Design review of the part built by this model. Coordinates are the model's own, in mm. Face numbers are marked on the shaded views. A direction names the side the tool comes from. Round coordinates to 2 decimals unless told otherwise and drop trailing zeros. Loops run counter-clockwise (first coordinate to the right, second up) from the corner with the lowest first, then second, coordinate; pieces in that order, holes last. Notation, with made-up numbers: M -40,-16 L 3,-16 A34 cw 3,18 Z; hole C 48,54 d2. An arc over 180 degrees is marked long. One line per item, written item: value. Start each with the question number.
Item 1: We need section D-D (y = -20.5). Write out the cut boundary in (x, z) (3 decimals), then the cut area to 3 significant figures.
Item 2: We need section A-A (z = -1.25). Write out the cut boundary in (x, y).
Item 3: Clearance check with flat-ended pins moving along their axes: pin 1 (5 mm diameter, centred on x = -11.5, z = -11, fed in from +Y); pin 2 (2 mm diameter, centred on x = 15.24, z = -11.625, fed in from +Y). State where each tip first meets the part, or that it passes through.
Item 4: We need section C-C (x = 11). Write out the cut boundary in (y, z), then the cut area to 3 significant figures.
Item 5: For the marked faces 1, 2 and 3, list the 3-axis set-ups (+Z, -Z, +X, -X, +Y, -Y) from which the entire face can be reached by the end or side of a thin tool; tool diameter is ignored.
Item 6: We need section B-B (z = -8). Write out the cut boundary in (x, y).
Item 7: Mouldability with a two-part tool opening along Y and no side actions: class the marked faces 4, 5 and 6 as released by +Y, released by -Y, zero draft, split by the parting line, or undercut.
Item 8: For line 1 along Y through (x, z) = (-6.35, 0.7); line 2 along X through (y, z) = (-17, -8.5); line 3 along Y through (x, z) = (-11, 1.75), list the stretches that pass through material, from the lowest coordinate up.
from build123d import *
from OCP.BRepFilletAPI import BRepFilletAPI_MakeChamfer

# Parameters (mm, degrees)
SKETCH_1_W          = 38.1
SKETCH_1_H          = 48
EXTRUDE_1_DEPTH     = 3
SKETCH_2_R          = 0.4
CUT_EXTRUDE_1_DEPTH = 31.78802527
SKETCH_3_W          = 38.1
SKETCH_3_H          = 15
EXTRUDE_2_DEPTH     = 17
SKETCH_4_W          = 2.75
SKETCH_4_H          = 2.75
CUT_EXTRUDE_2_DEPTH = 4
CHAMFER_1_SIZE      = 1
CHAMFER_1_SIZE_2    = 4
SKETCH_5_R          = 0.8
CUT_EXTRUDE_5_DEPTH = 55.36821222
SKETCH_6_W          = 38.1
SKETCH_6_H          = 11
CUT_EXTRUDE_6_DEPTH = 10
CUT_EXTRUDE_7_REACH = 34.232
SKETCH_8_W          = 1.6
SKETCH_8_H          = 6.622641265


with BuildPart() as part:
    # 草圖1 → 填料-伸長1 (new body)
    with BuildSketch(Plane.XY):
        Rectangle(SKETCH_1_W, SKETCH_1_H)
    extrude(amount=EXTRUDE_1_DEPTH)

    # 草圖2 → 除料-伸長1 (cut, through all)
    with BuildSketch(Plane.XY.offset(3)):
        with Locations((-16.51, 19)):
            Circle(SKETCH_2_R)
        with Locations((-13.97, 19)):
            Circle(SKETCH_2_R)
        with Locations((-6.35, 19)):
            Circle(SKETCH_2_R)
        with Locations((-3.81, 19)):
            Circle(SKETCH_2_R)
        with Locations((3.81, 19)):
            Circle(SKETCH_2_R)
        with Locations((6.35, 19)):
            Circle(SKETCH_2_R)
        with Locations((13.97, 19)):
            Circle(SKETCH_2_R)
        with Locations((16.51, 19)):
            Circle(SKETCH_2_R)
    extrude(amount=-CUT_EXTRUDE_1_DEPTH, mode=Mode.SUBTRACT)

    # 草圖3 → 填料-伸長2 (add)
    with BuildSketch(Plane(origin=(0, 0, 0), x_dir=(-1, 0, 0), z_dir=(0, 0, -1))):
        with Locations((0, -16.5)):
            Rectangle(SKETCH_3_W, SKETCH_3_H)
    extrude(amount=EXTRUDE_2_DEPTH)

    # 草圖4 → 除料-伸長2 (cut)
    with BuildSketch(Plane(origin=(0, -9, 0), x_dir=(1, 0, 0), z_dir=(0, 1, 0))):
        with Locations((-15.24, 11.625)):
            Rectangle(SKETCH_4_W, SKETCH_4_H)
        with Locations((-5.08, 11.625)):
            Rectangle(SKETCH_4_W, SKETCH_4_H)
        with Locations((5.08, 11.625)):
            Rectangle(SKETCH_4_W, SKETCH_4_H)
        with Locations((15.24, 11.625)):
            Rectangle(SKETCH_4_W, SKETCH_4_H)
    extrude(amount=-CUT_EXTRUDE_2_DEPTH, mode=Mode.SUBTRACT)

    # 導角1
    chamfer_1_edges_1 = [part.edges().sort_by_distance(p)[0] for p in [
        (-15.24, -9, -13),
    ]]
    chamfer_1_side_1 = [part.faces().sort_by_distance(p)[0] for p in [
        (-15.24, -9, -13.02),
    ]]
    chamfer_1_edges_2 = [part.edges().sort_by_distance(p)[0] for p in [
        (-13.865, -9, -11.625),
    ]]
    chamfer_1_side_2 = [part.faces().sort_by_distance(p)[0] for p in [
        (-13.845, -9, -11.625),
    ]]
    chamfer_1_edges_3 = [part.edges().sort_by_distance(p)[0] for p in [
        (-16.615, -9, -11.625),
    ]]
    chamfer_1_side_3 = [part.faces().sort_by_distance(p)[0] for p in [
        (-16.635, -9, -11.625),
    ]]
    chamfer_1_edges_4 = [part.edges().sort_by_distance(p)[0] for p in [
        (-15.24, -9, -10.25),
    ]]
    chamfer_1_side_4 = [part.faces().sort_by_distance(p)[0] for p in [
        (-15.24, -9, -10.23),
    ]]
    chamfer_1_edges_5 = [part.edges().sort_by_distance(p)[0] for p in [
        (15.24, -9, -10.25),
    ]]
    chamfer_1_side_5 = [part.faces().sort_by_distance(p)[0] for p in [
        (15.24, -9, -10.23),
    ]]
    chamfer_1_edges_6 = [part.edges().sort_by_distance(p)[0] for p in [
        (13.865, -9, -11.625),
    ]]
    chamfer_1_side_6 = [part.faces().sort_by_distance(p)[0] for p in [
        (13.845, -9, -11.625),
    ]]
    chamfer_1_edges_7 = [part.edges().sort_by_distance(p)[0] for p in [
        (16.615, -9, -11.625),
    ]]
    chamfer_1_side_7 = [part.faces().sort_by_distance(p)[0] for p in [
        (16.635, -9, -11.625),
    ]]
    chamfer_1_edges_8 = [part.edges().sort_by_distance(p)[0] for p in [
        (15.24, -9, -13),
    ]]
    chamfer_1_side_8 = [part.faces().sort_by_distance(p)[0] for p in [
        (15.24, -9, -13.02),
    ]]
    chamfer_1_edges_9 = [part.edges().sort_by_distance(p)[0] for p in [
        (5.08, -9, -10.25),
    ]]
    chamfer_1_side_9 = [part.faces().sort_by_distance(p)[0] for p in [
        (5.08, -9, -10.23),
    ]]
    chamfer_1_edges_10 = [part.edges().sort_by_distance(p)[0] for p in [
        (6.455, -9, -11.625),
    ]]
    chamfer_1_side_10 = [part.faces().sort_by_distance(p)[0] for p in [
        (6.475, -9, -11.625),
    ]]
    chamfer_1_edges_11 = [part.edges().sort_by_distance(p)[0] for p in [
        (5.08, -9, -13),
    ]]
    chamfer_1_side_11 = [part.faces().sort_by_distance(p)[0] for p in [
        (5.08, -9, -13.02),
    ]]
    chamfer_1_edges_12 = [part.edges().sort_by_distance(p)[0] for p in [
        (3.705, -9, -11.625),
    ]]
    chamfer_1_side_12 = [part.faces().sort_by_distance(p)[0] for p in [
        (3.685, -9, -11.625),
    ]]
    chamfer_1_edges_13 = [part.edges().sort_by_distance(p)[0] for p in [
        (-5.08, -9, -10.25),
    ]]
    chamfer_1_side_13 = [part.faces().sort_by_distance(p)[0] for p in [
        (-5.08, -9, -10.23),
    ]]
    chamfer_1_edges_14 = [part.edges().sort_by_distance(p)[0] for p in [
        (-6.455, -9, -11.625),
    ]]
    chamfer_1_side_14 = [part.faces().sort_by_distance(p)[0] for p in [
        (-6.475, -9, -11.625),
    ]]
    chamfer_1_edges_15 = [part.edges().sort_by_distance(p)[0] for p in [
        (-5.08, -9, -13),
    ]]
    chamfer_1_side_15 = [part.faces().sort_by_distance(p)[0] for p in [
        (-5.08, -9, -13.02),
    ]]
    chamfer_1_edges_16 = [part.edges().sort_by_distance(p)[0] for p in [
        (-3.705, -9, -11.625),
    ]]
    chamfer_1_side_16 = [part.faces().sort_by_distance(p)[0] for p in [
        (-3.685, -9, -11.625),
    ]]
    chamfer_1 = BRepFilletAPI_MakeChamfer(part.part.solid().wrapped)
    for e in chamfer_1_edges_1:
        chamfer_1.Add(CHAMFER_1_SIZE - 0.0001, CHAMFER_1_SIZE_2 - 0.0001, e.wrapped, chamfer_1_side_1[0].wrapped)
    for e in chamfer_1_edges_2:
        chamfer_1.Add(CHAMFER_1_SIZE - 0.0001, CHAMFER_1_SIZE_2 - 0.0001, e.wrapped, chamfer_1_side_2[0].wrapped)
    for e in chamfer_1_edges_3:
        chamfer_1.Add(CHAMFER_1_SIZE - 0.0001, CHAMFER_1_SIZE_2 - 0.0001, e.wrapped, chamfer_1_side_3[0].wrapped)
    for e in chamfer_1_edges_4:
        chamfer_1.Add(CHAMFER_1_SIZE - 0.0001, CHAMFER_1_SIZE_2 - 0.0001, e.wrapped, chamfer_1_side_4[0].wrapped)
    for e in chamfer_1_edges_5:
        chamfer_1.Add(CHAMFER_1_SIZE - 0.0001, CHAMFER_1_SIZE_2 - 0.0001, e.wrapped, chamfer_1_side_5[0].wrapped)
    for e in chamfer_1_edges_6:
        chamfer_1.Add(CHAMFER_1_SIZE - 0.0001, CHAMFER_1_SIZE_2 - 0.0001, e.wrapped, chamfer_1_side_6[0].wrapped)
    for e in chamfer_1_edges_7:
        chamfer_1.Add(CHAMFER_1_SIZE - 0.0001, CHAMFER_1_SIZE_2 - 0.0001, e.wrapped, chamfer_1_side_7[0].wrapped)
    for e in chamfer_1_edges_8:
        chamfer_1.Add(CHAMFER_1_SIZE - 0.0001, CHAMFER_1_SIZE_2 - 0.0001, e.wrapped, chamfer_1_side_8[0].wrapped)
    for e in chamfer_1_edges_9:
        chamfer_1.Add(CHAMFER_1_SIZE - 0.0001, CHAMFER_1_SIZE_2 - 0.0001, e.wrapped, chamfer_1_side_9[0].wrapped)
    for e in chamfer_1_edges_10:
        chamfer_1.Add(CHAMFER_1_SIZE - 0.0001, CHAMFER_1_SIZE_2 - 0.0001, e.wrapped, chamfer_1_side_10[0].wrapped)
    for e in chamfer_1_edges_11:
        chamfer_1.Add(CHAMFER_1_SIZE - 0.0001, CHAMFER_1_SIZE_2 - 0.0001, e.wrapped, chamfer_1_side_11[0].wrapped)
    for e in chamfer_1_edges_12:
        chamfer_1.Add(CHAMFER_1_SIZE - 0.0001, CHAMFER_1_SIZE_2 - 0.0001, e.wrapped, chamfer_1_side_12[0].wrapped)
    for e in chamfer_1_edges_13:
        chamfer_1.Add(CHAMFER_1_SIZE - 0.0001, CHAMFER_1_SIZE_2 - 0.0001, e.wrapped, chamfer_1_side_13[0].wrapped)
    for e in chamfer_1_edges_14:
        chamfer_1.Add(CHAMFER_1_SIZE - 0.0001, CHAMFER_1_SIZE_2 - 0.0001, e.wrapped, chamfer_1_side_14[0].wrapped)
    for e in chamfer_1_edges_15:
        chamfer_1.Add(CHAMFER_1_SIZE - 0.0001, CHAMFER_1_SIZE_2 - 0.0001, e.wrapped, chamfer_1_side_15[0].wrapped)
    for e in chamfer_1_edges_16:
        chamfer_1.Add(CHAMFER_1_SIZE - 0.0001, CHAMFER_1_SIZE_2 - 0.0001, e.wrapped, chamfer_1_side_16[0].wrapped)
    add(Compound.cast(chamfer_1.Shape()), mode=Mode.REPLACE)  # a hair under: the kernel refuses the full size

    # 草圖5 → 除料-伸長5 (cut, through all)
    with BuildSketch(Plane.XZ.offset(24)):
        with Locations(Location((-15.24, -11.625, 0), (0, 0, 270))):
            Circle(SKETCH_5_R)
        with Locations(Location((-5.08, -11.625, 0), (0, 0, 270))):
            Circle(SKETCH_5_R)
        with Locations(Location((5.08, -11.625, 0), (0, 0, 270))):
            Circle(SKETCH_5_R)
        with Locations(Location((15.24, -11.625, 0), (0, 0, 270))):
            Circle(SKETCH_5_R)
    extrude(amount=-CUT_EXTRUDE_5_DEPTH, mode=Mode.SUBTRACT)

    # 草圖6 → 除料-伸長6 (cut)
    with BuildSketch(Plane.XY.offset(3)):
        with Locations((0, -16.5)):
            Rectangle(SKETCH_6_W, SKETCH_6_H)
    extrude(amount=-CUT_EXTRUDE_6_DEPTH, mode=Mode.SUBTRACT)

    # 草圖8 → 除料-伸長7 (cut, up to next)
    with BuildSketch(Plane.XY.offset(-7), mode=Mode.PRIVATE) as cut_extrude_7_sk1:
        with Locations((-15.24, -18.688679368)):
            Rectangle(SKETCH_8_W, SKETCH_8_H)
    cut_extrude_7_tool1 = extrude(cut_extrude_7_sk1.sketch, amount=-CUT_EXTRUDE_7_REACH, mode=Mode.PRIVATE) & part.part
    # 草圖8 → 除料-伸長7 (cut, up to next)
    with BuildSketch(Plane.XY.offset(-7), mode=Mode.PRIVATE) as cut_extrude_7_sk2:
        with Locations((-5.08, -18.688679368)):
            Rectangle(SKETCH_8_W, SKETCH_8_H)
    cut_extrude_7_tool2 = extrude(cut_extrude_7_sk2.sketch, amount=-CUT_EXTRUDE_7_REACH, mode=Mode.PRIVATE) & part.part
    # 草圖8 → 除料-伸長7 (cut, up to next)
    with BuildSketch(Plane.XY.offset(-7), mode=Mode.PRIVATE) as cut_extrude_7_sk3:
        with Locations((5.08, -18.688679368)):
            Rectangle(SKETCH_8_W, SKETCH_8_H)
    cut_extrude_7_tool3 = extrude(cut_extrude_7_sk3.sketch, amount=-CUT_EXTRUDE_7_REACH, mode=Mode.PRIVATE) & part.part
    # 草圖8 → 除料-伸長7 (cut, up to next)
    with BuildSketch(Plane.XY.offset(-7), mode=Mode.PRIVATE) as cut_extrude_7_sk4:
        with Locations((15.24, -18.688679368)):
            Rectangle(SKETCH_8_W, SKETCH_8_H)
    cut_extrude_7_tool4 = extrude(cut_extrude_7_sk4.sketch, amount=-CUT_EXTRUDE_7_REACH, mode=Mode.PRIVATE) & part.part
    add(cut_extrude_7_tool1.solids().sort_by_distance((-15.24, -18.688679, -7))[0], mode=Mode.SUBTRACT)
    add(cut_extrude_7_tool2.solids().sort_by_distance((-5.08, -18.688679, -7))[0], mode=Mode.SUBTRACT)
    add(cut_extrude_7_tool3.solids().sort_by_distance((5.08, -18.688679, -7))[0], mode=Mode.SUBTRACT)
    add(cut_extrude_7_tool4.solids().sort_by_distance((15.24, -18.688679, -7))[0], mode=Mode.SUBTRACT)


solid = part.part
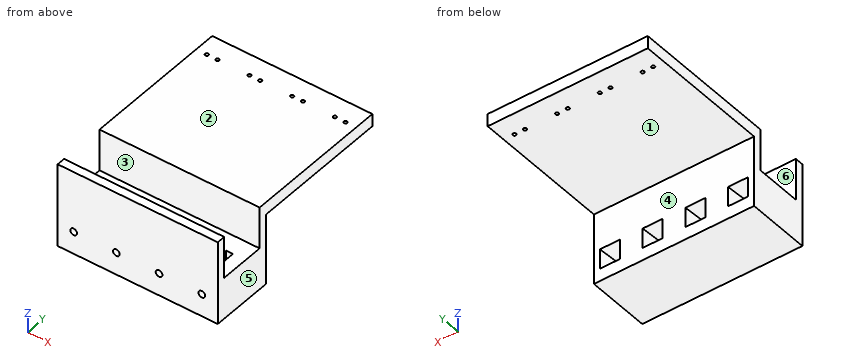
A:
1. outline: M -19.05,-17 L 19.05,-17 L 19.05,-7 L 16.04,-7 L 16.04,-11.625 A0.8 cw 14.44,-11.625 L 14.44,-7 L 5.88,-7 L 5.88,-11.625 A0.8 cw 4.28,-11.625 L 4.28,-7 L -4.28,-7 L -4.28,-11.625 A0.8 cw -5.88,-11.625 L -5.88,-7 L -14.44,-7 L -14.44,-11.625 A0.8 cw -16.04,-11.625 L -16.04,-7 L -19.05,-7 Z
1. area: 347 mm2
2. outline: M -19.05,-24 L 19.05,-24 L 19.05,-22 L -19.05,-22 Z; M -19.05,-11 L 19.05,-11 L 19.05,-9 L -19.05,-9 Z
3. pin 1: y = -9
3. pin 2: y = -13
4. outline: M -24,-17 L -9,-17 L -9,0 L 24,0 L 24,3 L -11,3 L -11,-7 L -22,-7 L -22,3 L -24,3 Z
4. area: 289 mm2
5. face 1: -Z, +X, -X, +Y
5. face 2: +Z, +X, -X, +Y, -Y
5. face 3: +Z, +X, -X
6. outline: M -19.05,-24 L 19.05,-24 L 19.05,-9 L -19.05,-9 Z; hole M -16.04,-22 L -14.44,-22 L -14.44,-15.38 L -16.04,-15.38 Z; hole M -5.88,-22 L -4.28,-22 L -4.28,-15.38 L -5.88,-15.38 Z; hole M 4.28,-22 L 5.88,-22 L 5.88,-15.38 L 4.28,-15.38 Z; hole M 14.44,-22 L 16.04,-22 L 16.04,-15.38 L 14.44,-15.38 Z
7. face 4: released by +Y
7. face 5: zero draft
7. face 6: undercut
8. line 1: -24 to -22, -11 to 18.6, 19.4 to 24
8. line 2: -19.05 to -16.04, -14.44 to -5.88, -4.28 to 4.28, 5.88 to 14.44, 16.04 to 19.05
8. line 3: -24 to -22, -11 to 24
